from build123d import *

# Parameters (mm, degrees)
SKETCH1_W           = 5.5
SKETCH1_H           = 7.612305333
SKETCH1_R           = 0.75
SKETCH1_R_2         = 8
BOSS_EXTRUDE1_DEPTH = 1.6


with BuildPart() as part:
    # Sketch1 → Boss-Extrude1 (new body)
    with BuildSketch(Plane.XY):
        with BuildLine():
            Line((5.5, 19.87), (-5.5, 19.87))
            Line((-5.5, 19.87), (-5.5, 11.882694667))
            Line((-5.5, 11.882694667), (-17.5, 11.882694667))
            Line((-17.5, 11.882694667), (-17.5, 8.632694667))
            Line((-17.5, 8.632694667), (-8.335261411, 8.632694667))
            ThreePointArc((-8.335261411, 8.632694667), (-11.956670593, -1.018836756), (-6.7545, -9.918504411))
            Line((-6.7545, -9.918504411), (-6.7545, -17.054889955))
            Line((-6.7545, -17.054889955), (6.7545, -17.054889955))
            Line((6.7545, -17.054889955), (6.7545, -9.918504411))
            ThreePointArc((6.7545, -9.918504411), (8.536775878, -8.433472453), (10, -6.633249581))
            Line((10, -6.633249581), (10, 6.633249581))
            ThreePointArc((10, 6.633249581), (9.221979067, 7.678222586), (8.335261411, 8.632694667))
            Line((8.335261411, 8.632694667), (17.5, 8.632694667))
            Line((17.5, 8.632694667), (17.5, 11.882694667))
            Line((17.5, 11.882694667), (5.5, 11.882694667))
            Line((5.5, 11.882694667), (5.5, 19.87))
        make_face()
        with Locations((0, 14.063847334)):
            Rectangle(SKETCH1_W, SKETCH1_H, mode=Mode.SUBTRACT)
        Polygon((-4.2545, -10.154889955), (4.2545, -10.154889955), (4.2545, -14.554889955), (1.25, -14.554889955), (1.25, -12.554889955), (-1.25, -12.554889955), (-1.25, -14.554889955), (-4.2545, -14.554889955), align=None, mode=Mode.SUBTRACT)
        with Locations((-15.18, 10.257694667)):
            Circle(SKETCH1_R, mode=Mode.SUBTRACT)
        Circle(SKETCH1_R_2, mode=Mode.SUBTRACT)
        with Locations((15.18, 10.257694667)):
            Circle(SKETCH1_R, mode=Mode.SUBTRACT)
    extrude(amount=BOSS_EXTRUDE1_DEPTH)


solid = part.part
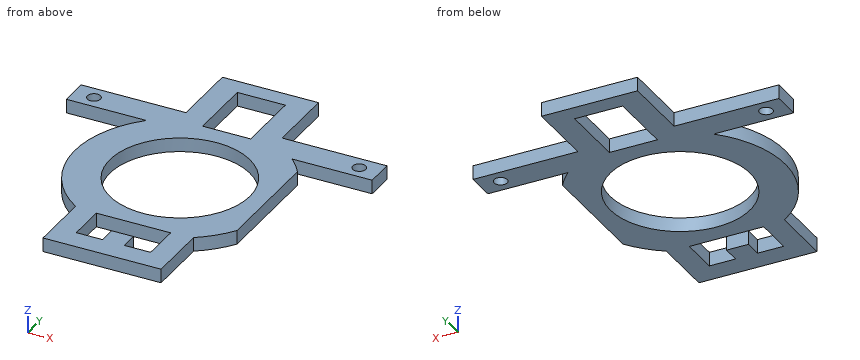
Read the model definition and answer for the solid it produces. Units are mm, in the model's axes. Coordinates: 2 decimals unless noted, no trailing zeros. Write each loop counter-clockwise with the first axis right and the second up, starting at its lowest first coordinate (ties: lowest second). Pieces come first, ordered by that corner, then holes. Notation, with made-up numbers: (64, -40) - (115, -40) arc R30 cw to (115, -1) - close; hole circle Ø2 at (51, -24.75). An arc over 180 degrees is marked (long way). One line per question, with ' | ' between items.
Q1. Find section C-C, the plane z = 0.35. State how many separate pieces and enclosed holes the cut face has, plus the area to 3 significant figures.
Result set:
separate pieces: 1 | enclosed holes: 5 | area: 396 mm^2
Q2. Find section A-A, the plane x = -15.18. Write down the section's boundary in (y, z).
Result set:
outline: (8.63, 0) - (9.51, 0) - (9.51, 1.6) - (8.63, 1.6) - close; (11.01, 0) - (11.88, 0) - (11.88, 1.6) - (11.01, 1.6) - close
Q3. Each of these flat-tipped pins is pushed along its axis until it touches: P1, Ø0.5, axis at y = 14.5, z = 0.5, coming from the -X side; P2, Ø0.8, axis at y = 2.5, z = 0.5, coming from the +X side; P3, Ø0.8, axis at x = -9.5, z = 1, coming from the +Y side; P4, Ø3, axis at x = -11, y = -10.5, coming from the +Z side. Where does it stop, or does it pass through?
Result set:
P1: x = -5.5 | P2: x = 10 | P3: y = 11.88 | P4: through
Q4. Find section B-B, the plane y = 0. Write down the section's boundary in (x, z).
Result set:
outline: (-12, 0) - (-8, 0) - (-8, 1.6) - (-12, 1.6) - close; (8, 0) - (10, 0) - (10, 1.6) - (8, 1.6) - close
Q5. Consider L1, parallel to Y at x = 0, z = 0.7; L2, parallel to Y at x = -10, z = 0.3; L3, parallel to Y at x = 15.18, z = 1.1. Determine where each line is inside the solid, lowest interval first. Write a range as [from, to].
Result set:
L1: [-17.05, -12.55], [-10.15, -8], [8, 10.26], [17.87, 19.87] | L2: [-6.63, 6.63], [8.63, 11.88] | L3: [8.63, 9.51], [11.01, 11.88]
Q6. Find section D-D, the plane y = -13. Write down the section's boundary in (x, z).
Result set:
outline: (-6.75, 0) - (-4.25, 0) - (-4.25, 1.6) - (-6.75, 1.6) - close; (-1.25, 0) - (1.25, 0) - (1.25, 1.6) - (-1.25, 1.6) - close; (4.25, 0) - (6.75, 0) - (6.75, 1.6) - (4.25, 1.6) - close
